Source: CAD feature listing. Evaluate the final solid. Frame: model axes, mm. Face numbers are marked on the shaded views. A direction names the side the tool comes from. Round coordinates to 2 decimals unless told otherwise and drop trailing zeros. Loops run counter-clockwise (first coordinate to the right, second up) from the corner with the lowest first, then second, coordinate; pieces in that order, holes last. Notation, with made-up numbers: (-3, -30.5) -> (4, -30.5) arc R30 ccw to (4, -6.5) -> close; hole circle Ø10 at (24.5, 43.25). An arc over 180 degrees is marked (long way). Return JSON: item names as keys, results as strings. Group by question number.
```python
from build123d import *

# Parameters (mm, degrees)
F0_W     = 78
F0_H     = 50
F1_DEPTH = 7.5
F3_DEPTH = 25
F4_W     = 78
F4_H     = 50
F4_W_2   = 70.5
F4_H_2   = 42.5
F5_DEPTH = 60


with BuildPart() as f1:
    # F0 (on Top) → F1 (new body)
    with BuildSketch(Plane.XY):
        Rectangle(F0_W, F0_H)
    extrude(amount=F1_DEPTH)

    # F2 (on face) → F3 (join)
    with BuildSketch(Plane.XY.offset(7.5)):
        with BuildLine():
            Line((-24.8326521918, 0), (-12.8640334502, 0))
            ThreePointArc((-12.8640334502, 0), (-18.848342821, 5.5663626469), (-24.8326521918, 0))
        make_face()
        with BuildLine():
            ThreePointArc((-12.848342821, -0.4336373531), (-12.8522667614, -0.2166767865), (-12.8640334502, 0))
            Line((-12.8640334502, 0), (-24.8326521918, 0))
            ThreePointArc((-24.8326521918, 0), (-19.0653033876, -6.4297134127), (-12.848342821, -0.4336373531))
        make_face()
        with BuildLine():
            Line((-6, 0), (0, 0))
            Line((0, 0), (6, 0))
            ThreePointArc((6, 0), (0, 6), (-6, 0))
        make_face()
        with BuildLine():
            Line((6, 0), (0, 0))
            Line((0, 0), (-6, 0))
            ThreePointArc((-6, 0), (0, -6), (6, 0))
        make_face()
        with BuildLine():
            ThreePointArc((25.1258996345, 0), (19.1332791001, 5.7025119665), (13.1406585656, 0))
            Line((13.1406585656, 0), (25.1258996345, 0))
        make_face()
        with BuildLine():
            Line((25.1258996345, 0), (13.1406585656, 0))
            ThreePointArc((13.1406585656, 0), (18.9844893267, -6.2956428834), (25.1332791001, -0.2974880335))
            ThreePointArc((25.1332791001, -0.2974880335), (25.13143395, -0.1486982602), (25.1258996345, 0))
        make_face()
    extrude(amount=F3_DEPTH)

    # F4 (on face) → F5 (join)
    with BuildSketch(Plane(origin=(0, 0, 0), x_dir=(1, 0, 0), z_dir=(0, 0, -1))):
        Rectangle(F4_W, F4_H)
        Rectangle(F4_W_2, F4_H_2, mode=Mode.SUBTRACT)
    extrude(amount=F5_DEPTH)


solid = f1.part
```
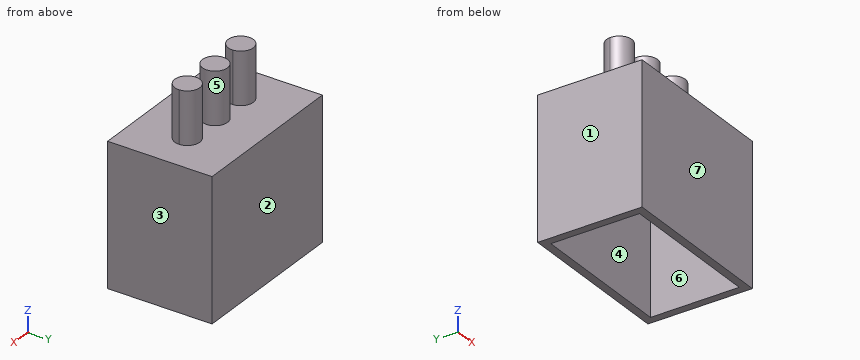
(1) Cut plane A-A (z = -23.5). Return loops of the section in (x, y).
(2) Cut plane D-D (x = 0). Return loops of the section in (y, z).
(3) Set-up query: the marked faces 5, 6 and 7. Return all of +Z, -Z, +X, -X, +Y, -Y with unobstructed straight access to the full face (end or side cutting, diameter ignored); none if empty.
(4) Cut plane B-B (x = 9). Return loops of the section in (y, z), and give its area (3 significant figures).
(5) Pin query (flat end, axial travel): pin 1 (6 mm diameter, centred on x = -28.5, y = -6, fed in from +Z); pin 2 (8 mm diameter, centred on x = 23, y = -16.5, fed in from -Z). Return the tip coordinate at first contact, or that it passes through.
(6) Cut plane C-C (y = 8.5). Return loops of the section in (x, z).
(7) Ray query, line 1 (Y direction, x = -2.5, z = -54); line 2 (X direction, y = -21, z = -51.5); line 3 (Z direction, x = 13, y = 10). Return the intervals inside material, ascending.
(8) Mould query, pull axis X, two halves, no side actions, for the marked faces 1, 2, 3 and 4. Classes: released by +X, released by -X, zero draft, split by the parting line, or undercut.
Answers follow:
{
 "1": {"outline": "(-39, -25) -> (39, -25) -> (39, 25) -> (-39, 25) -> close; hole (-35.25, -21.25) -> (35.25, -21.25) -> (35.25, 21.25) -> (-35.25, 21.25) -> close"},
 "2": {"outline": "(-25, -60) -> (-21.25, -60) -> (-21.25, 0) -> (21.25, 0) -> (21.25, -60) -> (25, -60) -> (25, 7.5) -> (6, 7.5) -> (6, 32.5) -> (-6, 32.5) -> (-6, 7.5) -> (-25, 7.5) -> close"},
 "3": {"face 5": "+Z", "face 6": "-Z", "face 7": "+Z, -Z, +X, -X, -Y"},
 "4": {"outline": "(-25, -60) -> (-21.25, -60) -> (-21.25, 0) -> (21.25, 0) -> (21.25, -60) -> (25, -60) -> (25, 7.5) -> (-25, 7.5) -> close", "area": "825 mm^2"},
 "5": {"pin 1": "z = 7.5", "pin 2": "z = 0"},
 "6": {"outline": "(-39, -60) -> (-35.25, -60) -> (-35.25, 0) -> (35.25, 0) -> (35.25, -60) -> (39, -60) -> (39, 7.5) -> (-39, 7.5) -> close"},
 "7": {"line 1": "-25 to -21.25, 21.25 to 25", "line 2": "-39 to -35.25, 35.25 to 39", "line 3": "0 to 7.5"},
 "8": {"face 1": "released by -X", "face 2": "zero draft", "face 3": "released by +X", "face 4": "undercut"}
}
